CAD build for the part. Positions are in the model's coordinates, mm. A direction names the side the tool comes from. Round coordinates to 2 decimals unless told otherwise and drop trailing zeros. Write each loop counter-clockwise with the first axis right and the second up, starting at its lowest first coordinate (ties: lowest second). Pieces come first, ordered by that corner, then holes. Notation, with made-up numbers: (18, 82.25) - (54, 82.25) arc R6 ccw to (54, 92.25) - close; hole circle Ø11 at (62, 69). An arc over 180 degrees is marked (long way). Answer in a Markdown table with one row per item.
```python
from build123d import *

# Parameters (mm, degrees)
F0_W     = 25
F0_H     = 40
F0_R     = 6.25
F1_DEPTH = 3.2
F2_R     = 3.25
F2_W     = 25
F2_H     = 40
F3_DEPTH = 35
F4_W     = 15
F4_H     = 46.4
F4_R     = 2.25
F5_DEPTH = 5
F6_SIZE  = 2
F7_R     = 3.25
F7_R_2   = 2.25
F8_DEPTH = 3.2


with BuildPart() as f1:
    # F0 (on Top) → F1 (new body)
    with BuildSketch(Plane.XY):
        Rectangle(F0_W, F0_H)
        Circle(F0_R, mode=Mode.SUBTRACT)
    extrude(amount=F1_DEPTH)

    # F2 (on face) → F3 (join)
    with BuildSketch(Plane.XY.offset(3.2)):
        with BuildLine():
            Line((15.7, -23.2), (15.7, 23.2))
            Line((15.7, 23.2), (7.5, 23.2))
            Line((7.5, 23.2), (7.5, 27.5))
            ThreePointArc((7.5, 27.5), (0, 35), (-7.5, 27.5))
            Line((-7.5, 27.5), (-7.5, 23.2))
            Line((-7.5, 23.2), (-15.7, 23.2))
            Line((-15.7, 23.2), (-15.7, -23.2))
            Line((-15.7, -23.2), (-7.5, -23.2))
            Line((-7.5, -23.2), (-7.5, -27.5))
            ThreePointArc((-7.5, -27.5), (0, -35), (7.5, -27.5))
            Line((7.5, -27.5), (7.5, -23.2))
            Line((7.5, -23.2), (15.7, -23.2))
        make_face()
        with Locations((0, -27.5)):
            Circle(F2_R, mode=Mode.SUBTRACT)
        Rectangle(F2_W, F2_H, mode=Mode.SUBTRACT)
        with BuildLine():
            ThreePointArc((0, 24.25), (-2.2980970389, 29.7980970389), (3.25, 27.5))
            ThreePointArc((3.25, 27.5), (2.2980970389, 25.2019029611), (0, 24.25))
        make_face(mode=Mode.SUBTRACT)
    extrude(amount=-F3_DEPTH)

    # F4 (on face) → F5 (join)
    with BuildSketch(Plane.XY.offset(3.2)):
        with Locations((-23.2, 0)):
            Rectangle(F4_W, F4_H)
        with Locations((-23.2, -13.2)):
            Circle(F4_R, mode=Mode.SUBTRACT)
        with Locations((-23.2, 13.2)):
            Circle(F4_R, mode=Mode.SUBTRACT)
    extrude(amount=-F5_DEPTH)

    # F6
    f6_edges = [f1.edges().sort_by_distance(p)[0] for p in [
        (15.7, 23.2, -14.3),
        (-15.7, 23.2, -16.8),
        (-15.7, -23.2, -16.8),
        (15.7, -23.2, -14.3),
        (-30.7, 23.2, 0.7),
        (-30.7, -23.2, 0.7),
    ]]
    chamfer(f6_edges, length=F6_SIZE)

    # F7 (on face) → F8 (join)
    with BuildSketch(Plane(origin=(0, 0, -31.8), x_dir=(1, 0, 0), z_dir=(0, 0, -1))):
        with Locations((0, -27.5)):
            Circle(F7_R)
        with Locations((0, -27.5)):
            Circle(F7_R_2, mode=Mode.SUBTRACT)
        with Locations((0, 27.5)):
            Circle(F7_R)
        with Locations((0, 27.5)):
            Circle(F7_R_2, mode=Mode.SUBTRACT)
    extrude(amount=-F8_DEPTH)


solid = f1.part
```
Q1. Flat gauge pins, fed straight in: pin 1 (5 mm diameter, centred on x = -23.5, y = -8.5, fed in from -Z); pin 2 (5 mm diameter, centred on x = 9, z = -15.5, fed in from +Y); pin 3 (2 mm diameter, centred on y = 26.5, z = -13.5, fed in from +X). Where does each tip first touch, or does it go through?
Computed:
| item | result |
|---|---|
| pin 1 | stops at z = -1.8 |
| pin 2 | stops at y = 31.24 |
| pin 3 | stops at x = 7.5 |
Q2. Pull direction X, two halves, no side cores. Call faces 1 (the flat face through (11, -23.2, -14)), 2 (the flat face through (-12.5, 0, -16)), 3 (the flat face through (7.5, -25, -14)): released by +X, released by -X, zero draft, split by the parting line, or undercut.
Computed:
| item | result |
|---|---|
| face 1 | zero draft |
| face 2 | undercut |
| face 3 | released by +X |
Q3. Saw through at A-A on y = 0. List the corners of the cut face in (x, z).
Computed:
| item | result |
|---|---|
| outline | (-30.7, -1.8) - (-15.7, -1.8) - (-15.7, -31.8) - (-12.5, -31.8) - (-12.5, 0) - (-6.25, 0) - (-6.25, 3.2) - (-30.7, 3.2) - close; (6.25, 0) - (12.5, 0) - (12.5, -31.8) - (15.7, -31.8) - (15.7, 3.2) - (6.25, 3.2) - close |
Q4. Saw through at C-C on z = -22.5. List the corners of the cut face in (x, y), then the cut area to 3 significant figures.
Computed:
| item | result |
|---|---|
| outline | (-15.7, -21.2) - (-13.7, -23.2) - (-7.5, -23.2) - (-7.5, -27.5) arc R7.5 ccw to (7.5, -27.5) - (7.5, -23.2) - (13.7, -23.2) - (15.7, -21.2) - (15.7, 21.2) - (13.7, 23.2) - (7.5, 23.2) - (7.5, 27.5) arc R7.5 ccw to (-7.5, 27.5) - (-7.5, 23.2) - (-13.7, 23.2) - (-15.7, 21.2) - close; hole (-12.5, -20) - (12.5, -20) - (12.5, 20) - (-12.5, 20) - close; hole circle Ø6.5 at (0, -27.5); hole circle Ø6.5 at (0, 27.5) |
| area | 688 mm2 |
Q5. 3-axis set-ups, long thin cutter, end or side, ignore diameter. For faces 4 (the flat face through (-13.5, -23.2, -10.2)), 5 (the flat face through (-13.5, 23.2, -10.2)), 6 (the flat face through (-1, 30, -28.6)): which of +Z, -Z, +X, -X, +Y, -Y reach the whole face in a straight line?
Computed:
| item | result |
|---|---|
| face 4 | +Z, -Z, -X, -Y |
| face 5 | +Z, -Z, -X, +Y |
| face 6 | +Z |
Q6. Saw through at B-B on x = -23.2. List the corners of the cut face in (y, z), then the cut area to 3 significant figures.
Computed:
| item | result |
|---|---|
| outline | (-23.2, -1.8) - (-15.45, -1.8) - (-15.45, 3.2) - (-23.2, 3.2) - close; (-10.95, -1.8) - (10.95, -1.8) - (10.95, 3.2) - (-10.95, 3.2) - close; (15.45, -1.8) - (23.2, -1.8) - (23.2, 3.2) - (15.45, 3.2) - close |
| area | 187 mm2 |
Q7. Saw through at D-D on y = -10. List the corners of the cut face in (x, z), then the cut area to 3 significant figures.
Computed:
| item | result |
|---|---|
| outline | (-30.7, -1.8) - (-15.7, -1.8) - (-15.7, -31.8) - (-12.5, -31.8) - (-12.5, 0) - (12.5, 0) - (12.5, -31.8) - (15.7, -31.8) - (15.7, 3.2) - (-30.7, 3.2) - close |
| area | 379 mm2 |
Q8. Drill centre lines: line 1 (Y direction, x = -23.2, z = 0.55); line 2 (Y direction, x = 0, z = -13); line 3 (X direction, y = 11, z = -13). Where is each one in solid material? Low to high.
Computed:
| item | result |
|---|---|
| line 1 | y = -23.2 to -15.45, -10.95 to 10.95, 15.45 to 23.2 |
| line 2 | y = -35 to -30.75, -24.25 to -20, 20 to 24.25, 30.75 to 35 |
| line 3 | x = -15.7 to -12.5, 12.5 to 15.7 |
